```python
from build123d import *

# Parameters (mm, degrees)
F0_W     = 203.2
F0_H     = 101.6
F1_DEPTH = 25.4
F2_R     = 12.7
F3_DEPTH = 25.4
F4_W     = 38.1
F4_H     = 50.8
F6_W     = 25.4
F6_H     = 12.7
F8_R     = 2.54
F9_SIZE  = 2.54


with BuildPart() as f1:
    # F0 (on Front) → F1 (new body)
    with BuildSketch(Plane.XZ):
        Rectangle(F0_W, F0_H)
    extrude(amount=F1_DEPTH)

    # F2 (on Front) → F3 (cut)
    with BuildSketch(Plane.XZ):
        with Locations((-63.5, 31.75)):
            Circle(F2_R)
        with Locations((-63.5, -31.75)):
            Circle(F2_R)
        with Locations((63.5, 31.75)):
            Circle(F2_R)
        with Locations((63.5, -31.75)):
            Circle(F2_R)
    extrude(amount=F3_DEPTH, mode=Mode.SUBTRACT)

    # F4 (on Top) → F5 (revolve)
    with BuildSketch(Plane.XY):
        with Locations((-19.05, 25.4)):
            Rectangle(F4_W, F4_H)
    revolve(axis=Axis((0, 25.4, 0), (0, -1, 0)))

    # F6 (on Top) → F7 (revolve, cut)
    with BuildSketch(Plane.XY):
        with Locations((-31.75, 25.7521334298)):
            Rectangle(F6_W, F6_H)
    revolve(axis=Axis((0, 67.0673400164, 0), (0, 1, 0)), mode=Mode.SUBTRACT)

    # F8
    f8_edges = [f1.edges().sort_by_distance(p)[0] for p in [
        (38.1, 0, 0),
        (19.05, 19.402133, 0),
        (19.05, 32.102133, 0),
    ]]
    fillet(f8_edges, radius=F8_R)

    # F9
    f9_edges = [f1.edges().sort_by_distance(p)[0] for p in [
        (38.1, 50.8, 0),
        (38.1, 32.102133, 0),
        (38.1, 19.402133, 0),
        (-101.6, 0, 0),
        (0, 0, -50.8),
        (0, 0, 50.8),
        (101.6, 0, 0),
    ]]
    chamfer(f9_edges, length=F9_SIZE)


solid = f1.part
```
Design review of the part built by this model. Coordinates are the model's own, in mm. A direction names the side the tool comes from. Coordinates: 2 decimals unless noted, no trailing zeros. Order: outer loops, then holes, each group sorted by start corner. A loop starts at its lowest first (then second) coordinate and runs counter-clockwise, first axis right, second up. Notation, with made-up numbers: M 52,17.25 L 110,17.25 A15 cw 110,32.25 Z; hole C -30,-27 d10. An arc over 180 degrees is marked long. Answer as a JSON object with one key per item and string values. Group by question number.
1) Mouldability with a two-part tool opening along Z and no side actions: class faces 1 (the cylindrical face through (-51.768, -12.522, -36.614)), 2 (the conical face through (7.74, 32.26, -34.87)), 3 (the cylindrical face through (-57.64, -12.522, 20.483)), 4 (the flat face through (-1, -14, 50.8)) as pulls with the +Z half, pulls with the -Z half, needs draft (parallel to the pull), parting line crosses it, or undercut.
2) Add section A-A, the plane x = 63.5. Write out the cut boundary in (y, z).
3) For pin 1 (1 mm diameter, centred on y = 34.5, z = 9.5, fed in from +X); pin 2 (2 mm diameter, centred on y = 25.5, z = 8, fed in from +X); pin 3 (12 mm diameter, centred on x = -57, z = -30, fed in from +Y); pin 4 (1 mm diameter, centred on y = -2.5, z = -2.5, fed in from -X), all flat-tipped, find the tip position at first contact; note any pin that passes through.
4) Tool access review of faces 5 (the flat face through (0, 32.102, -23)), 6 (the flat face through (-1, -25.4, 1)), 7 (the cylindrical face through (30.235, 9.801, 23.183)): name each direction out of +Z, -Z, +X, -X, +Y, -Y from which nothing blocks a thin tool from reaching the whole face with its end or side.
5) Add section C-C, the plane y = 26.5. Write out the cut boundary in (x, z).
6) Wall thickness on L1, parallel to Z at x = -63.5, y = -13.25; L2, parallel to X at y = -7.5, z = 40; L3, parallel to Y at x = -92.5, z = -46.5: over which ranges is each line inside the solid? List them lowest first.
Computed values:
{
 "1": {"face 1": "undercut", "face 2": "parting line crosses it", "face 3": "undercut", "face 4": "pulls with the +Z half"},
 "2": {"outline": "M -25.4,-50.8 L -2.54,-50.8 L 0,-48.26 L 0,-44.45 L -25.4,-44.45 Z; M -25.4,-19.05 L 0,-19.05 L 0,19.05 L -25.4,19.05 Z; M -25.4,44.45 L 0,44.45 L 0,48.26 L -2.54,50.8 L -25.4,50.8 Z"},
 "3": {"pin 1": "stops at x = 37.02", "pin 2": "stops at x = 17.72", "pin 3": "stops at y = 0", "pin 4": "stops at x = -101.6"},
 "4": {"face 5": "none", "face 6": "+Z, -Z, +X, -X, -Y", "face 7": "+Y"},
 "5": {"outline": "C 0,0 d38.1"},
 "6": {"L1": "z = -50.8 to -44.45, -19.05 to 19.05, 44.45 to 50.8", "L2": "x = -101.6 to -73.16, -53.84 to 53.84, 73.16 to 101.6", "L3": "y = -25.4 to 0"}
}
